from build123d import *

# Parameters (mm, degrees)
EXTRUDE_1_DEPTH     = 5
EXTRUDE_2_DEPTH     = 20
CUT_EXTRUDE_1_DEPTH = 166.263426081
CUT_EXTRUDE_2_DEPTH = 2.5
SKETCH_6_W          = 21
SKETCH_6_H          = 5
EXTRUDE_3_DEPTH     = 2.5


with BuildPart() as part:
    # 스케치1 → 보스-돌출1 (new body)
    with BuildSketch(Plane(origin=(0, 0, 0), x_dir=(1, 0, 0), z_dir=(0, 1, 0))):
        with BuildLine():
            Line((0, 95), (0, 116))
            Line((0, 116), (116, 116))
            Line((116, 116), (116, 0))
            Line((116, 0), (95, 0))
            ThreePointArc((95, 0), (67.175144213, 67.175144213), (0, 95))
        make_face()
    extrude(amount=EXTRUDE_1_DEPTH)

    # 스케치2 → 보스-돌출2 (add)
    with BuildSketch(Plane(origin=(0, 5, 0), x_dir=(1, 0, 0), z_dir=(0, 1, 0))):
        with BuildLine():
            Line((97, 0), (100, 0))
            ThreePointArc((100, 0), (70.710678119, 70.710678119), (0, 100))
            Line((0, 100), (0, 97))
            ThreePointArc((0, 97), (68.589357775, 68.589357775), (97, 0))
        make_face()
    extrude(amount=EXTRUDE_2_DEPTH)

    # 스케치3 → 컷-돌출1 (cut, through all)
    with BuildSketch(Plane(origin=(0, 5, 0), x_dir=(1, 0, 0), z_dir=(0, 1, 0))):
        with BuildLine():
            Line((20, 105), (84.852813742, 105))
            ThreePointArc((84.852813742, 105), (87.267323582, 103.002010829), (89.634803308, 100.948511807))
            Line((89.634803308, 100.948511807), (67.66435687, 78.978065369))
            ThreePointArc((67.66435687, 78.978065369), (45.325930989, 93.603204966), (20, 102.058806577))
            Line((20, 102.058806577), (20, 105))
        make_face()
        with BuildLine():
            Line((105, 84.852813742), (105, 20))
            Line((105, 20), (102.058806577, 20))
            ThreePointArc((102.058806577, 20), (93.603204966, 45.325930989), (78.978065369, 67.66435687))
            Line((78.978065369, 67.66435687), (100.948511807, 89.634803308))
            ThreePointArc((100.948511807, 89.634803308), (103.002010829, 87.267323582), (105, 84.852813742))
        make_face()
    extrude(amount=-CUT_EXTRUDE_1_DEPTH, mode=Mode.SUBTRACT)

    # 스케치5 → 컷-돌출2 (cut)
    with BuildSketch(Plane.XZ):
        Polygon((0, -95), (0, -116), (5, -116), (5, -94.868329805), align=None)
    extrude(amount=-CUT_EXTRUDE_2_DEPTH, mode=Mode.SUBTRACT)

    # 스케치6 → 보스-돌출3 (add)
    with BuildSketch(Plane(origin=(0, 0, 0), x_dir=(1, 0, 0), z_dir=(0, 1, 0))):
        with Locations((105.5, -2.5)):
            Rectangle(SKETCH_6_W, SKETCH_6_H)
    extrude(amount=EXTRUDE_3_DEPTH)


solid = part.part
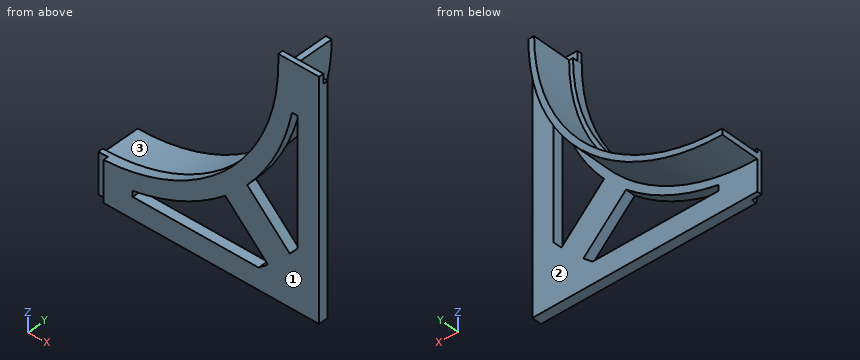
Verification items for the finished model (mm, model axes). Face numbers are marked on the shaded views. A direction names the side the tool comes from. Coordinates: 2 decimals unless noted, no trailing zeros. Loops run counter-clockwise (first coordinate to the right, second up) from the corner with the lowest first, then second, coordinate; pieces in that order, holes last. Notation, with made-up numbers: M -26.5,-0.5 L 4.5,-0.5 A31 ccw 4.5,27.5 Z; hole C 28,-16 d8. An arc over 180 degrees is marked long. One line per item, written item: value.
1. Section check A-A on x = 71. Record the cut outline in (y, z), plus the area to 3 significant figures.
Answers follow:
outline: M 0,-116 L 5,-116 L 5,-105 L 0,-105 Z; M 0,-82.31 L 5,-82.31 L 5,-70.42 L 25,-70.42 L 25,-66.09 L 5,-66.09 L 5,-63.12 L 0,-63.12 Z
area: 238 mm^2
2. Set-up check for the marked faces 1, 2 and 3: record each of +Z, -Z, +X, -X, +Y, -Y from which the full face is reachable in a straight line by a thin tool's end or side.
Answers follow:
face 1: +Z, -Z, +X, -X, -Y
face 2: -Z, +X, +Y
face 3: +Z, -X, +Y
3. Section check B-B on z = -74. Record the cut outline in (x, y).
Answers follow:
outline: M 59.57,0 L 85.31,0 L 85.31,5 L 67.26,5 L 67.26,25 L 62.71,25 L 62.71,5 L 59.57,5 Z; M 105,0 L 116,0 L 116,5 L 105,5 Z
4. Gauge pin test, flat ends, axial feed: P1, Ø1, axis at y = 18.5, z = -37.5, coming from the +X side; P2, Ø1.5, axis at x = 108, z = 2.5, coming from the +Y side; P3, Ø5, axis at y = 11, z = -66, coming from the -X side; P4, Ø5, axis at x = 63, z = -100.5, coming from the +Y side. Record the tip position at first contact, or that the pin passes through.
Answers follow:
P1: x = 92.9
P2: y = 2.5
P3: x = 68.68
P4: through
5. Material ranges on line 1 along Y through (x, z) = (34, -110); line 2 along X through (y, z) = (1.5, -35.5); line 3 along X through (y, z) = (2.25, -40), recorded low to high. Write a range as from..to.
Answers follow:
line 1: 0..5
line 2: 88.12..97.75, 105..116
line 3: 86.17..96, 105..116
6. Section check D-D on x = 9.5. Record the cut outline in (y, z), plus the area to 3 significant figures.
Answers follow:
outline: M 0,-116 L 5,-116 L 5,-99.55 L 25,-99.55 L 25,-96.53 L 5,-96.53 L 5,-94.52 L 0,-94.52 Z
area: 168 mm^2
7. Section check C-C on y = 15.25. Record the cut outline in (x, z), plus the area to 3 significant figures.
Answers follow:
outline: M 0,-100 A100 ccw 100,0 L 97,0 A97 cw 0,-97 Z
area: 464 mm^2
